Verification items for the finished model (mm, model axes). Face numbers are marked on the shaded views. A direction names the side the tool comes from. Round coordinates to 2 decimals unless told otherwise and drop trailing zeros. Write each loop counter-clockwise with the first axis right and the second up, starting at its lowest first coordinate (ties: lowest second). Pieces come first, ordered by that corner, then holes. Notation, with made-up numbers: (79, -7) - (90, -7) arc R18 cw to (90, 10) - close; hole circle Ø11 at (-13, 43.5). An arc over 180 degrees is marked (long way). Answer as a JSON object with one key per item and string values.
```python
from build123d import *

# Parameters (mm, degrees)
BOSS_EXTRUDE1_DEPTH = 40
BOSS_EXTRUDE1_DRAFT = -15
SHELL1_T            = -10


with BuildPart() as part:
    # Sketch1 → Boss-Extrude1 (with draft: the straight prism first)
    with BuildSketch(Plane(origin=(0, 0, 0), x_dir=(1, 0, 0), z_dir=(0, 1, 0))):
        with BuildLine():
            Line((-109.029856613, -113.081906669), (109.029856613, -113.081906669))
            Line((109.029856613, -113.081906669), (109.029856613, 113.081906669))
            ThreePointArc((109.029856613, 113.081906669), (0, 152.401411753), (-109.029856613, 113.081906669))
            Line((-109.029856613, 113.081906669), (-109.029856613, -113.081906669))
        make_face()
    extrude(amount=BOSS_EXTRUDE1_DEPTH)
    # Boss-Extrude1: the draft: its side faces are tilted about the plane it starts from
    boss_extrude1_sides = [part.faces().sort_by_distance(p)[0] for p in [
        (0, 20, 113.081906669),
        (109.029856613, 20, 0),
        (0, 20, -152.401411753),
        (-109.029856613, 20, 0),
    ]]
    draft(boss_extrude1_sides, Plane(origin=(0, 0, 0), x_dir=(1, 0, 0), z_dir=(0, 1, 0)), BOSS_EXTRUDE1_DRAFT)

    # Shell1
    shell1_openings = [part.faces().sort_by_distance(p)[0] for p in [
        (0, 40, -12.878837242),
    ]]
    offset(amount=SHELL1_T, openings=shell1_openings, kind=Kind.INTERSECTION)


solid = part.part
```
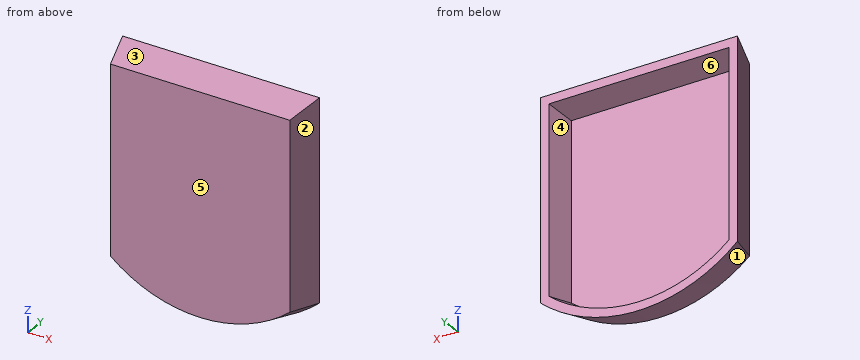
Q1. Gauge pin test, flat ends, axial feed: P1, Ø6, axis at x = 83, z = -54.5, coming from the -Y side; P2, Ø6, axis at x = -79.5, y = 22, coming from the +Z side; P3, Ø1.5, axis at x = 46.5, y = 5, coming from the -Z side; P4, Ø12, axis at x = -56.5, y = 33, coming from the +Z side. Record the tip position at first contact, or that the pin passes through.
Geometry check:
{"P1": "stops at y = 0", "P2": "stops at z = 119.78", "P3": "stops at z = -147.64", "P4": "stops at z = 123.53"}
Q2. Set-up check for the marked faces 5 and 6: record each of +Z, -Z, +X, -X, +Y, -Y from which the full face is reachable in a straight line by a thin tool's end or side.
Geometry check:
{"face 5": "+Z, -Z, +X, -X, -Y", "face 6": "+Y"}
Q3. Release check for a two-part mould opening along X. For the marked faces 1, 2, 3 and 4 record: released by +X, released by -X, zero draft, split by the parting line, or undercut.
Geometry check:
{"face 1": "split by the parting line", "face 2": "released by +X", "face 3": "zero draft", "face 4": "undercut"}
Q4. Section check A-A, the plane y = 19. Record the cut outline in (x, z), then the cut area to 3 significant figures.
Geometry check:
{"outline": "(-114.12, -115.45) arc R175.92 ccw to (114.12, -115.45) - (114.12, 118.17) - (-114.12, 118.17) - close; hole (-103.77, -110.59) arc R165.56 ccw to (103.77, -110.59) - (103.77, 107.82) - (-103.77, 107.82) - close", "area": "9,380 mm2"}
Q5. Material ranges on line 1 along Y through (x, z) = (-68, 30.5); line 2 along X through (y, z) = (37, -102); line 3 along X through (y, z) = (38, -80.5), recorded low to high. Write a range as [from, to].
Geometry check:
{"line 1": "y = [0, 10]", "line 2": "x = [-118.94, -108.59], [108.59, 118.94]", "line 3": "x = [-119.21, -108.86], [108.86, 119.21]"}
Q6. Section check B-B, the plane z = -47.5. Record the cut outline in (x, y).
Geometry check:
{"outline": "(-119.75, 40) - (-109.03, 0) - (109.03, 0) - (119.75, 40) - (109.4, 40) - (101.36, 10) - (-101.36, 10) - (-109.4, 40) - close"}
